Job drawing, mm, ordinate dimensions from the low corner. One solid piece. A direction names the side the tool comes from. Coordinates: 2 decimals unless noted, no trailing zeros. Write each loop counter-clockwise with the first axis right and the second up, starting at its lowest first coordinate (ties: lowest second). Pieces come first, ordered by that corner, then holes.
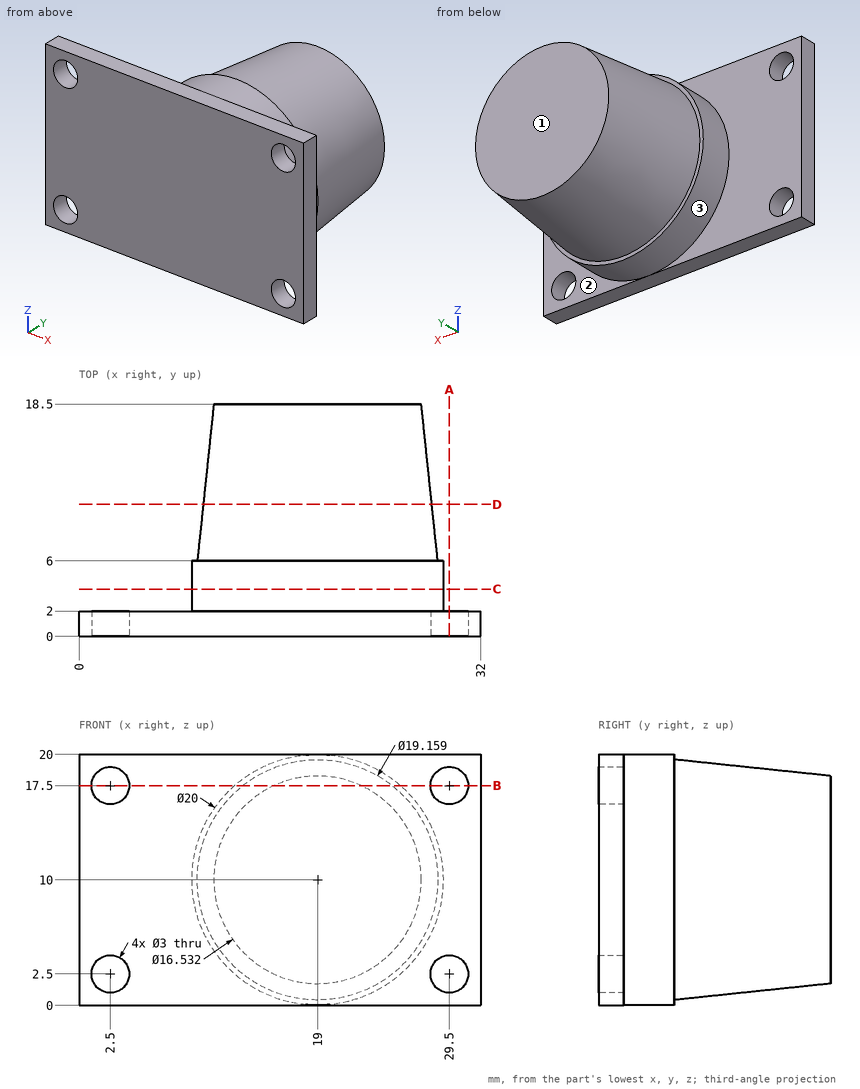
1. Saw through at C-C on y = 3.75. List the corners of the cut face in (x, z), plus the area to 3 significant figures.
Computed values:
outline: circle Ø20 at (19, 10)
area: 314 mm2
2. 3-axis set-ups, long thin cutter, end or side, ignore diameter. For the marked faces 1, 2 and 3: which of +Z, -Z, +X, -X, +Y, -Y reach the whole face in a straight line?
Computed values:
face 1: +Z, -Z, +X, -X, +Y
face 2: +X, +Y
face 3: +Y
3. Saw through at B-B on z = 17.5. State how many separate pieces and enclosed holes the cut face has, plus the area to 3 significant figures.
Computed values:
separate pieces: 3
enclosed holes: 0
area: 225 mm2
4. Saw through at A-A on x = 29.5. List the corners of the cut face in (y, z).
Computed values:
outline: (0, 0) - (2, 0) - (2, 1) - (0, 1) - close; (0, 4) - (2, 4) - (2, 16) - (0, 16) - close; (0, 19) - (2, 19) - (2, 20) - (0, 20) - close
5. Saw through at D-D on y = 10.5. List the corners of the cut face in (x, z).
Computed values:
outline: circle Ø18.21 at (19, 10)
6. Flat gauge pins, fed straight in: pin 1 (3.5 mm diameter, centred on x = 2.5, z = 17.5, fed in from +Y); pin 2 (2 mm diameter, centred on y = 16.5, z = 7, fed in from +X); pin 3 (10 mm diameter, centred on x = 13, y = 8, fed in from +Z). Where does each tip first touch, or does it go through?
Computed values:
pin 1: stops at y = 2
pin 2: stops at x = 27.26
pin 3: stops at z = 19.9
7. Probe line 1 along X through (y, z) = (0.7, 2.5); line 2 along Y through (x, z) = (31.5, 1.5); line 3 along Z through (x, y) = (15, 10). List the from-to ranges inside material, lowest first.
Computed values:
line 1: x = 0 to 1, 4 to 28, 31 to 32
line 2: y = 0 to 2
line 3: z = 1.76 to 18.24
